from build123d import *

# Parameters (mm, degrees)
BOSS_EXTRUDE1_DEPTH      = 30
CUT_EXTRUDE4_DEPTH       = 40
CUT_EXTRUDE4_DEPTH_BACK  = 40
SKETCH7_W                = 30
SKETCH7_H                = 66.933951842
BOSS_EXTRUDE2_DEPTH      = 15
BOSS_EXTRUDE2_DEPTH_BACK = 15
SKETCH12_W               = 30
SKETCH12_H               = 41
CUT_EXTRUDE7_DEPTH       = 20
SKETCH13_W               = 40
SKETCH13_H               = 41
BOSS_EXTRUDE4_DEPTH      = 10
SKETCH15_W               = 8
SKETCH15_H               = 8
BOSS_EXTRUDE5_DEPTH      = 20
BOSS_EXTRUDE5_DEPTH_BACK = 10
SKETCH17_R               = 1
CUT_EXTRUDE9_DEPTH       = 30
SKETCH18_R               = 24.806306278
CUT_EXTRUDE10_DEPTH      = 20
SKETCH19_R               = 4
SKETCH19_R_2             = 1.5
CUT_EXTRUDE11_DEPTH      = 30
SKETCH20_W               = 56
SKETCH20_H               = 100
BOSS_EXTRUDE6_DEPTH      = 10
SKETCH24_W               = 50
SKETCH24_H               = 80
CUT_EXTRUDE13_DEPTH      = 20
CUT_EXTRUDE14_DEPTH      = 70
SKETCH30_W               = 6
SKETCH30_H               = 20
CUT_EXTRUDE15_DEPTH      = 30


with BuildPart() as part:
    # Sketch2 → Boss-Extrude1 (new body)
    with BuildSketch(Plane(origin=(0, 0, 0), x_dir=(0, 0, -1), z_dir=(1, 0, 0))):
        with BuildLine():
            Line((-15, 35), (15, 35))
            Line((15, 35), (15, -35))
            ThreePointArc((15, -35), (0, -90.980762114), (-15, -35))
            Line((-15, -35), (-15, 35))
        make_face()
    extrude(amount=BOSS_EXTRUDE1_DEPTH)

    # Sketch6 → Cut-Extrude4 (cut, two sides)
    with BuildSketch(Plane.XY) as cut_extrude4_sk:
        Polygon((15, 35), (30, -15.145060683), (30, -44.036502572), (15, -91.543130052), (48.566296189, -91.543130052), (48.566296189, 35), align=None)
    extrude(amount=CUT_EXTRUDE4_DEPTH, mode=Mode.SUBTRACT)
    extrude(cut_extrude4_sk.sketch, amount=-CUT_EXTRUDE4_DEPTH_BACK, mode=Mode.SUBTRACT)

    # Sketch7 → Boss-Extrude2 (add, two sides)
    with BuildSketch(Plane.XY) as boss_extrude2_sk:
        with Locations((15, 1.533024079)):
            Rectangle(SKETCH7_W, SKETCH7_H)
    extrude(amount=BOSS_EXTRUDE2_DEPTH)
    extrude(boss_extrude2_sk.sketch, amount=-BOSS_EXTRUDE2_DEPTH_BACK)

    # Sketch12 → Cut-Extrude7 (cut)
    with BuildSketch(Plane.XY.offset(15)):
        with Locations((15, 14.5)):
            Rectangle(SKETCH12_W, SKETCH12_H)
    extrude(amount=-CUT_EXTRUDE7_DEPTH, mode=Mode.SUBTRACT)

    # Sketch13 → Boss-Extrude4 (add)
    with BuildSketch(Plane.XY.offset(-5)):
        with Locations((15, 14.596252504)):
            Rectangle(SKETCH13_W, SKETCH13_H)
    extrude(amount=-BOSS_EXTRUDE4_DEPTH)

    # Sketch15 → Boss-Extrude5 (add, two sides)
    with BuildSketch(Plane.XY.offset(-5)) as boss_extrude5_sk:
        with Locations((39, 29.096252504)):
            Rectangle(SKETCH15_W, SKETCH15_H)
        with Locations((-9, 29.096252504)):
            Rectangle(SKETCH15_W, SKETCH15_H)
    extrude(amount=BOSS_EXTRUDE5_DEPTH)
    extrude(boss_extrude5_sk.sketch, amount=-BOSS_EXTRUDE5_DEPTH_BACK)

    # Sketch17 → Cut-Extrude9 (cut)
    with BuildSketch(Plane(origin=(0, 33.096252504, 0), x_dir=(1, 0, 0), z_dir=(0, 1, 0))):
        with Locations((39, 0)):
            Circle(SKETCH17_R)
        with Locations((39, -10)):
            Circle(SKETCH17_R)
        with Locations((-9, 0)):
            Circle(SKETCH17_R)
        with Locations((-9, -10)):
            Circle(SKETCH17_R)
    extrude(amount=-CUT_EXTRUDE9_DEPTH, mode=Mode.SUBTRACT)

    # Sketch18 → Cut-Extrude10 (cut)
    with BuildSketch(Plane(origin=(30, 0, 0), x_dir=(0, 0, -1), z_dir=(1, 0, 0))):
        with Locations((0, -60.980762114)):
            Circle(SKETCH18_R)
    extrude(amount=-CUT_EXTRUDE10_DEPTH, mode=Mode.SUBTRACT)

    # Sketch19 → Cut-Extrude11 (cut)
    with BuildSketch(Plane(origin=(30, 0, 0), x_dir=(0, 0, -1), z_dir=(1, 0, 0))):
        with Locations((0, -60.980762114)):
            Circle(SKETCH19_R)
        with Locations((0, -52.980762114)):
            Circle(SKETCH19_R_2)
        with Locations((0, -68.980762114)):
            Circle(SKETCH19_R_2)
    extrude(amount=-CUT_EXTRUDE11_DEPTH, mode=Mode.SUBTRACT)

    # Sketch20 → Boss-Extrude6 (add)
    with BuildSketch(Plane.XY.offset(-5)):
        with Locations((15, 85.096252504)):
            Rectangle(SKETCH20_W, SKETCH20_H)
    extrude(amount=-BOSS_EXTRUDE6_DEPTH)

    # Sketch24 → Cut-Extrude13 (cut)
    with BuildSketch(Plane.XY.offset(-5)):
        with Locations((12, 95.096252504)):
            Rectangle(SKETCH24_W, SKETCH24_H)
    extrude(amount=-CUT_EXTRUDE13_DEPTH, mode=Mode.SUBTRACT)

    # Sketch25 → Cut-Extrude14 (cut)
    with BuildSketch(Plane(origin=(43, 0, 0), x_dir=(0, 0, -1), z_dir=(1, 0, 0))):
        Polygon((10, 50.096252504), (8, 50.096252504), (8, 46.596252504), (3.330307532, 46.596252504), (3.330307532, 43.596252504), (8, 43.596252504), (8, 40.096252504), (10, 40.096252504), align=None)
    extrude(amount=-CUT_EXTRUDE14_DEPTH, mode=Mode.SUBTRACT)

    # Sketch30 → Cut-Extrude15 (cut)
    with BuildSketch(Plane.XY.offset(-5)):
        with Locations((-10, 45.096252504)):
            Rectangle(SKETCH30_W, SKETCH30_H)
    extrude(amount=-CUT_EXTRUDE15_DEPTH, mode=Mode.SUBTRACT)


solid = part.part
Model file for the job. Use its own axes, mm. A direction names the side the tool comes from. Give positions to 0.01 mm unless a question says otherwise; leave off trailing zeros. Write each loop counter-clockwise with the first axis right and the second up, starting at its lowest first coordinate (ties: lowest second). Pieces come first, ordered by that corner, then holes. Notation, with made-up numbers: M -19,-29 L 36,-29 A29 ccw 36,2 Z; hole C 17.25,7 d6. An arc over 180 degrees is marked long. One line per item, written item: value. Start each with the question number.
Q1. Drop flat-ended pins along their axis: pin 1 Ø4 at (x, y) = (21, 36) entering from +Z; pin 2 Ø10 at (x, z) = (19, 6.5) entering from -Y; pin 3 Ø8 at (x, z) = (22, -11) entering from +Y. Give the stop position or say it passes through.
Q2. Saw through at A-A, the plane x = 32.5. Write the cut outline in (y, z).
Q3. Probe probe 1 along X at (y, z) = (27, 10); probe 2 along Y at (x, z) = (2, 0); probe 3 along Z at (x, y) = (39, 30.5). List the from-to ranges inside material, lowest first. Write a range as [from, to].
Q4. Saw through at B-B, the plane x = 4. Write the cut outline in (y, z).
Q5. Saw through at C-C, the plane y = -29. Write the cut outline in (x, z), plus the area to 3 significant figures.
Q6. 3-axis set-ups, long thin cutter, end or side, ignore diameter. For faces 1 (the flat face through (-7, 45, -11)), 2 (the cylindrical face through (17.918, -36.386, 3.229)), 3 (the flat face through (37, 25.096, 0)), 4 (the flat face through (39, 35.096, -10)): which of +Z, -Z, +X, -X, +Y, -Y reach the whole face in a straight line?
Q7. Two-plate mould, pull along X, no slides. Class faces 5 (the flat face through (-11, 25.096, 0)), 6 (the flat face through (-5, 9, -10)), 7 (the flat face through (-5, 29, 5)), 8 (the flat face through (35, 29, 5)): +X half, -X half, draft (parallel to the pull), parting line (faces both ways), or undercut.
Output values:
1. pin 1: stops at z = -5
1. pin 2: stops at y = -90.81
1. pin 3: stops at y = 55.1
2. outline: M -5.9,-15 L 55.1,-15 L 55.1,-5 L 46.6,-5 L 46.6,-8 L 50.1,-8 L 50.1,-10 L 40.1,-10 L 40.1,-8 L 43.6,-8 L 43.6,-5 L -5.9,-5 Z
3. probe 1: x = [-13, -10], [-8, -5], [35, 38], [40, 43]
3. probe 2: y = [-90.98, -70.48], [-67.48, -64.98], [-56.98, -54.48], [-51.48, -6]
3. probe 3: z = [-15, -1], [1, 9], [11, 15]
4. outline: M -35,-15 L 55.1,-15 L 55.1,-5 L 46.6,-5 L 46.6,-8 L 50.1,-8 L 50.1,-10 L 40.1,-10 L 40.1,-8 L 43.6,-8 L 43.6,-5 L -6,-5 L -6,15 L -35,15 A30 ccw long Z; hole C -68.98,0 d3; hole C -60.98,0 d8; hole C -52.98,0 d3
5. outline: M 0,-15 L 30,-15 L 30,15 L 0,15 Z
5. area: 900 mm²
6. face 1: +Z, -Z, -X, +Y
6. face 2: +X
6. face 3: +Z, -Z, +X, -Y
6. face 4: +Z, -Z, +X
7. face 5: draft
7. face 6: -X half
7. face 7: undercut
7. face 8: undercut
